Input: part model. Units: mm. Frame: model coordinates. Face numbers are marked on the shaded views. A direction names the side the tool comes from. Give positions to 0.01 mm unless a question says otherwise; leave off trailing zeros. Loops run counter-clockwise (first coordinate to the right, second up) from the corner with the lowest first, then second, coordinate; pieces in that order, holes last. Notation, with made-up numbers: M 89.5,1 L 102.5,1 A18 ccw 102.5,17 Z; hole C -5.5,25.5 d4. An arc over 180 degrees is marked long. Answer as a JSON object with one key per item and string values. Group by question number.
1) Section query A-A on y = 4.5. Return loops of the section in (x, z).
2) Ray query, L1, parallel to Z at x = 13.5, y = 2; L2, parallel to X at y = -34.5, z = 2; L3, parallel to Z at x = 13.5, y = 20.5. Return the intervals inside material, ascending.
3) First-contact query: P1, Ø5, axis at x = 5, z = -2.5, coming from the -Y side; P2, Ø8, axis at x = 14, y = -0.5, coming from the +Z side; P3, Ø3.5, axis at x = 11.5, y = 21.5, coming from the +Z side. Flat tips, straight axial feed; report the tip coordinate or a pass-through.
4) Draft query along Y for the marked faces 1, 2 and 3. Return one class per face: +Y half, -Y half, draft (parallel to the pull), parting line (faces both ways), or undercut.
5) Access query for the marked faces 4, 5 and 6. Directions: +Z, -Z, +X, -X, +Y, -Y. A direction counts if a zero-diameter tool reaches every point of the face in a straight line with its end or side. Return the directions, or none.
from build123d import *

# Parameters (mm, degrees)
SKETCH1_W           = 16.85
SKETCH1_H           = 8.9
BOSS_EXTRUDE1_DEPTH = 19
SKETCH2_W           = 7.5
SKETCH2_H           = 2.2
SKETCH2_W_2         = 4.6
BOSS_EXTRUDE2_DEPTH = 6.2
CHAMFER1_SIZE       = 0.5
SKETCH3_RX          = 5.9
SKETCH3_RY          = 4.45
BOSS_EXTRUDE3_DEPTH = 13.4
CHAMFER2_SIZE       = 2
SKETCH4_R           = 2.75


with BuildPart() as part:
    # Sketch1 → Boss-Extrude1 (new body)
    with BuildSketch(Plane(origin=(0, 0, 0), x_dir=(1, 0, 0), z_dir=(0, 1, 0))):
        with Locations((8.425, 4.45)):
            Rectangle(SKETCH1_W, SKETCH1_H)
    extrude(amount=BOSS_EXTRUDE1_DEPTH)

    # Sketch2 → Boss-Extrude2 (add)
    with BuildSketch(Plane(origin=(0, 19, 0), x_dir=(1, 0, 0), z_dir=(0, 1, 0))):
        with Locations((6.025, 4.45)):
            Rectangle(SKETCH2_W, SKETCH2_H)
        with Locations((12.275, 4.45)):
            Rectangle(SKETCH2_W_2, SKETCH2_H)
    extrude(amount=BOSS_EXTRUDE2_DEPTH)

    # Chamfer1
    chamfer1_edges = [part.edges().sort_by_distance(p)[0] for p in [
        (2.275, 22.1, -5.55),
        (9.775, 22.1, -5.55),
    ]]
    chamfer(chamfer1_edges, length=CHAMFER1_SIZE)

    # Sketch3 → Boss-Extrude3 (add)
    with BuildSketch(Plane.XZ):
        with Locations(Location((8.425, -4.45), (0, 0, 180))):
            Ellipse(SKETCH3_RX, SKETCH3_RY)
    extrude(amount=BOSS_EXTRUDE3_DEPTH)

    # Chamfer2
    chamfer2_edges = [part.edges().sort_by_distance(p)[0] for p in [
        (16.85, 0, -4.45),
        (0, 0, -4.45),
    ]]
    chamfer(chamfer2_edges, length=CHAMFER2_SIZE)

    # Sweep2: sweep along a path in Sketch6
    with BuildLine(Plane(origin=(0, 0, 0), x_dir=(0, 0, -1), z_dir=(1, 0, 0))) as sweep2_path:
        ThreePointArc((4.45, -13.4), (-6.679942315, -40.270057685), (-33.55, -51.4))
    # Sketch4 → Sweep2 (sweep)
    with BuildSketch(Plane.XZ.offset(13.4)):
        with Locations((8.425, -4.45)):
            Circle(SKETCH4_R)
    sweep(path=sweep2_path.line)


solid = part.part
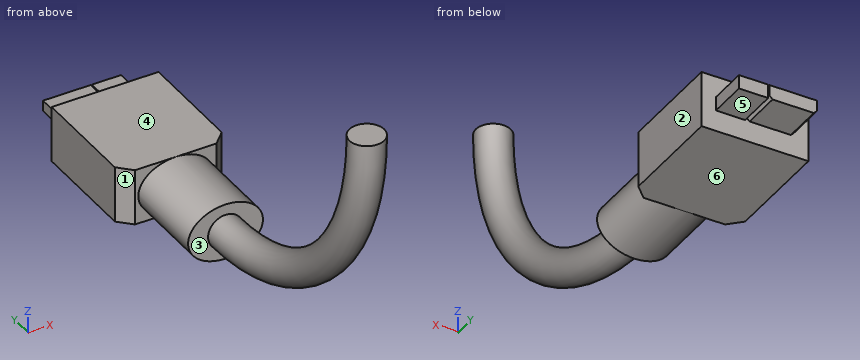
Output:
{
 "1": {"outline": "M 0,-8.9 L 16.85,-8.9 L 16.85,0 L 0,0 Z"},
 "2": {"L1": "z = -8.9 to 0", "L2": "x = 5.68 to 11.17", "L3": "z = -5.55 to -3.35"},
 "3": {"P1": "stops at y = -34.39", "P2": "stops at z = 0", "P3": "stops at z = -3.35"},
 "4": {"face 1": "-Y half", "face 2": "draft", "face 3": "undercut"},
 "5": {"face 4": "+Z, +X, -X, +Y", "face 5": "-Z, +X, -X, +Y", "face 6": "-Z, +X, -X, +Y, -Y"}
}
